Design review of the part built by this model. Coordinates are the model's own, in mm. A direction names the side the tool comes from. Coordinates: 2 decimals unless noted, no trailing zeros. Order: outer loops, then holes, each group sorted by start corner. A loop starts at its lowest first (then second) coordinate and runs counter-clockwise, first axis right, second up.
Autodesk Inventor part; units mm, degrees
ref_plane "YZ Plane" through (0, 0, 0) normal (1, 0, 0) x (0, 1, 0)
ref_plane "XZ Plane" through (0, 0, 0) normal (0, 1, 0) x (-1, 0, 0)
ref_plane "XY Plane" through (0, 0, 0) normal (0, 0, 1) x (1, 0, 0)
sketch "Sketch1" plane through (0, 0, 0) normal (0, 1, 0) x (-1, 0, 0)
  line L0 (-9.525, 11.43) -> (9.525, 11.43)
  line L1 (9.525, 11.43) -> (9.525, -11.43)
  line L2 (9.525, -11.43) -> (-9.525, -11.43)
  line L3 (-9.525, -11.43) -> (-9.525, 11.43)
  line L4 (-9.525, 11.43) -> (9.525, -11.43) construction
  line L5 (9.525, 11.43) -> (-9.525, -11.43) construction
  point P0 (0, 0)
  dimension "d0" = 19.05
  dimension "d1" = 22.86
extrude "Extrusion1" add sketch "Sketch1" along normal blind 20.32
sketch "Sketch2" plane through (0, 20.32, 0) normal (0, 1, 0) x (1, 0, 0)
  circle A0 centre (0, 0) radius 9.144
  dimension "d4" = 18.288
extrude "Extrusion2" add sketch "Sketch2" along normal blind 10.16
sketch "Sketch3" plane through (0, 30.48, 0) normal (0, 1, 0) x (1, 0, 0)
  line L0 (-9.525, 11.43) -> (-9.525, -11.43)
  line L1 (-9.525, 5.4993) -> (0, 10.9985)
  line L2 (0, 10.9985) -> (9.525, 5.4993)
  line L3 (9.525, 5.4993) -> (9.525, -5.4993)
  line L4 (9.525, -5.4993) -> (0, -10.9985)
  line L5 (0, -10.9985) -> (-9.525, -5.4993)
  line L6 (-9.525, -5.4993) -> (-9.525, 5.4993)
  point P0 (0, 0)
  point P1 (0, 0)
  point P2 (-9.525, 0)
extrude "Extrusion3" add sketch "Sketch3" along normal blind 8.255
chamfer "Chamfer1" distance 0.7937 angle 45 13 edges at (9.525, 10.16, 11.43) (-9.525, 10.16, 11.43) (9.525, 10.16, -11.43) (-9.525, 10.16, -11.43) (0, 0, -11.43) (9.525, 0, 0) (0, 0, 11.43) (-9.525, 0, 0) (9.525, 20.32, 0) (0, 20.32, 11.43) (-9.525, 20.32, 0) (0, 20.32, -11.43) (-9.144, 30.48, 0)
sketch "Sketch4" plane through (0, 38.735, 0) normal (0, 1, 0) x (1, 0, 0)
  circle A0 centre (0, 0) radius 7.0485
  dimension "d12" = 14.097
extrude "Extrusion4" add sketch "Sketch4" along normal blind 13.5128
sketch "Sketch5" plane through (0, 52.2478, 0) normal (0, 1, 0) x (1, 0, 0)
  circle A0 centre (0, 0) radius 8.255
  dimension "d15" = 16.51
extrude "Extrusion5" add sketch "Sketch5" along normal blind 1.524
sketch "Sketch6" plane through (0, 53.7718, 0) normal (0, 1, 0) x (1, 0, 0)
  line L0 (0, -10.9985) -> (9.525, -5.4993)
  line L1 (0, -10.9985) -> (-9.525, -5.4993)
  line L2 (-9.525, -5.4993) -> (-9.525, 5.4993)
  line L3 (-9.525, 5.4993) -> (0, 10.9985)
  line L4 (0, 10.9985) -> (9.525, 5.4993)
  line L5 (9.525, 5.4993) -> (9.525, -5.4993)
  line L6 (9.525, -5.4993) -> (0, -10.9985)
  point P0 (0, 0)
  point P1 (0, 0)
extrude "Extrusion6" add sketch "Sketch6" along normal blind 6.35
sketch "Sketch7" plane through (0, 60.1218, 0) normal (0, 1, 0) x (1, 0, 0)
  circle A0 centre (0, 0) radius 8.255
  dimension "d20" = 16.51
extrude "Extrusion7" add sketch "Sketch7" along normal blind 1.524
sketch "Sketch8" plane through (0, 61.6458, 0) normal (0, 1, 0) x (1, 0, 0)
  circle A0 centre (0, 0) radius 9.525
  dimension "d23" = 19.05
extrude "Extrusion8" add sketch "Sketch8" along normal blind 16.002
sketch "Sketch9" plane through (0, 77.6478, 0) normal (0, 1, 0) x (1, 0, 0)
  circle A0 centre (0, 0) radius 10.4775
  dimension "d26" = 20.955
extrude "Extrusion9" add sketch "Sketch9" along normal blind 12.7
thread "Thread1"
chamfer "Chamfer2" distance 0.3969 angle 45 4 edges at (-8.255, 52.2478, 0) (-8.255, 53.7718, 0) (-8.255, 60.1218, 0) (-8.255, 61.6458, 0)
chamfer "Chamfer3" distance 0.3969 angle 45 1 edges at (-10.4775, 77.6478, 0)
properties part number "NeedleValveCAD"
1. Mouldability with a two-part tool opening along Y and no side actions: class faces 1 (the flat face through (-4, 60.122, 8)), 2 (the flat face through (0, 0, 0)), 3 (the flat face through (-9, 30.48, 5)), 4 (the cylindrical face through (-1.36, 84.11, 10.39)) as pulls with the +Y half, pulls with the -Y half, needs draft (parallel to the pull), parting line crosses it, or undercut.
2. Add section B-B (y = 43.5). Give the boundary of the cut face in (x, z).
3. Add section A-A (y = 17). Give the boundary of the cut face in (x, z) (3 decimals).
4. Insertion check: pin 1 (7 mm diameter, centred on y = 36.5, z = 1, fed in from -X) (3 decimals); pin 2 (1 mm diameter, centred on y = 68, z = 0.5, fed in from +X) (3 decimals); pin 3 (10 mm diameter, centred on x = -3, z = -7.5, fed in from -Y); pin 4 (2 mm diameter, centred on x = -2, y = 32, fed in from +Z). Each pin has a flat end and moves straight along its axis. Give the tip position at first contact, or say it passes through.
5. For faces 5 (the cylindrical face through (7.874, 60.879, 2.48)), 6 (the flat face through (-4.83, 34.34, -8.21)), 7 (the flat face through (4.696, 56.902, 8.287)), list the 3-axis set-ups (+Z, -Z, +X, -X, +Y, -Y) from which the entire face can be reached by the end or side of a thin tool; tool diameter is ignored.
6. To check wall thickness, follow line 1 (Y direction, x = 8, z = -3.5) (3 decimals); line 2 (Y direction, x = -8.75, z = 5.5) (3 decimals); line 3 (Y direction, x = 0.75, z = 8.25) (3 decimals). State the ranges of each line that lie inside material, in increasing order.
Solution:
1. face 1: undercut
1. face 2: pulls with the -Y half
1. face 3: undercut
1. face 4: needs draft
2. outline: circle Ø14.1 at (0, 0)
3. outline: (-9.525, -10.636) - (-8.731, -11.43) - (8.731, -11.43) - (9.525, -10.636) - (9.525, 10.636) - (8.731, 11.43) - (-8.731, 11.43) - (-9.525, 10.636) - close
4. pin 1: stops at x = -9.525
4. pin 2: stops at x = 9.525
4. pin 3: stops at y = 0
4. pin 4: stops at z = 10.42
5. face 5: none
5. face 6: -Z, -X
5. face 7: +Z, +X
6. line 1: y = 0 to 38.735, 53.772 to 60.122, 61.646 to 90.348
6. line 2: y = 0.019 to 20.301, 30.48 to 38.735, 53.772 to 60.122, 77.902 to 90.348
6. line 3: y = 0 to 38.735, 53.404 to 60.49, 61.278 to 90.348
